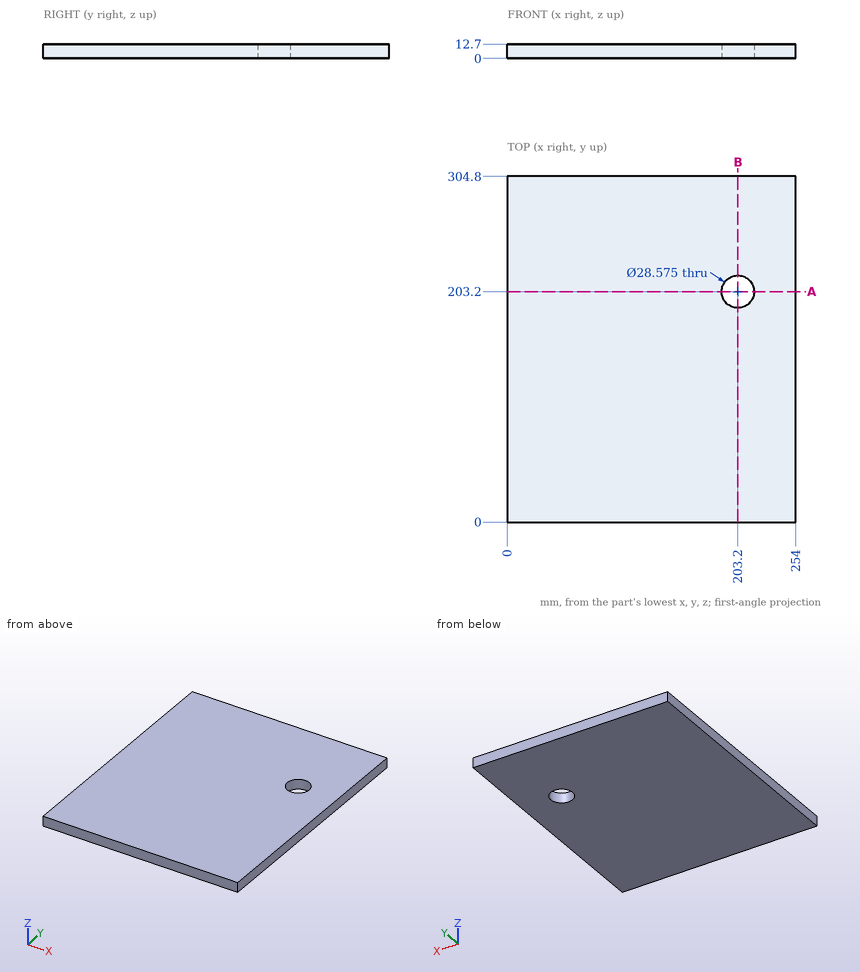
For this review, use the dimensioned drawing (mm, ordinates from the lowest corner) and the shaded views. Give positions to 0.01 mm unless a question says otherwise; leave off trailing zeros. Write each loop counter-clockwise with the first axis right and the second up, starting at its lowest first coordinate (ties: lowest second). Pieces come first, ordered by that corner, then holes. Notation, with made-up numbers: M -32,89 L 18,89 A16 cw 18,108 Z; hole C 83,-40 d2. An arc over 180 degrees is marked long. Answer as a JSON object with one key per item and string values. Group by question number.
1) Clearance check with a flat-ended pin moving along its axis: pin 1 Ø8 at (x, y) = (89, 265) entering from -Z. State where the tip first meets the part, or that it passes through.
2) For line 1 along X through (y, z) = (203.2, 10); line 2 along Y through (x, z) = (203.2, 9.25); line 3 along Y through (x, z) = (200, 7.75), list the stretches that pass through material, from the lowest coordinate up.
3) We need section A-A (y = 203.2). Give the boundary of the cut face in (x, z), and give its area (3 significant figures).
4) We need section B-B (x = 203.2). Give the boundary of the cut face in (y, z).
Answer key:
{
 "1": {"pin 1": "stops at z = 0"},
 "2": {"line 1": "x = 0 to 188.91, 217.49 to 254", "line 2": "y = 0 to 188.91, 217.49 to 304.8", "line 3": "y = 0 to 189.28, 217.12 to 304.8"},
 "3": {"outline": "M 0,0 L 188.91,0 L 188.91,12.7 L 0,12.7 Z; M 217.49,0 L 254,0 L 254,12.7 L 217.49,12.7 Z", "area": "2,860 mm²"},
 "4": {"outline": "M 0,0 L 188.91,0 L 188.91,12.7 L 0,12.7 Z; M 217.49,0 L 304.8,0 L 304.8,12.7 L 217.49,12.7 Z"}
}
